Here's how the part is built. I have some questions about the finished solid (model axes, mm). Face numbers are marked on the shaded views. A direction names the side the tool comes from. Round coordinates to 2 decimals unless told otherwise and drop trailing zeros. Order: outer loops, then holes, each group sorted by start corner. A loop starts at its lowest first (then second) coordinate and runs counter-clockwise, first axis right, second up. Notation, with made-up numbers: (76, 33.25) - (128, 33.25) arc R4 ccw to (128, 37.25) - close; hole circle Ø11 at (-28, 18). An arc over 180 degrees is marked (long way). Answer as a JSON object with one key per item and string values.
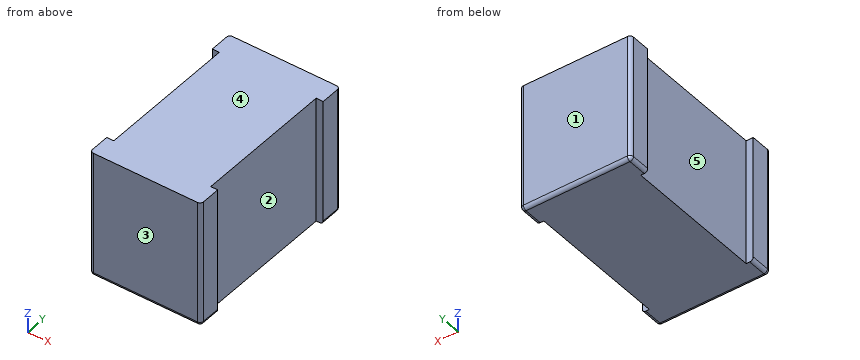
```python
from build123d import *

# Parameters (mm, degrees)
SKETCH_W        = 7.9
SKETCH_H        = 13.2
PAD_DEPTH       = 9.5
SKETCH004_W     = 10
SKETCH004_H     = 9.5
POCKET_DEPTH    = 0.5
POCKET001_DEPTH = 0.5
FILLET001_R     = 0.25


with BuildPart() as part:
    # Sketch → Pad (new body)
    with BuildSketch(Plane.XY):
        Rectangle(SKETCH_W, SKETCH_H)
    extrude(amount=PAD_DEPTH)

    # Sketch004 → Pocket (cut)
    with BuildSketch(Plane.YZ.offset(3.95)):
        with Locations((0, 4.75)):
            Rectangle(SKETCH004_W, SKETCH004_H)
    pocket = extrude(amount=-POCKET_DEPTH, mode=Mode.SUBTRACT)

    # Mirrored: Pocket across YZ
    add(pocket.mirror(Plane.YZ), mode=Mode.SUBTRACT)

    # Sketch005 → Pocket001 (cut)
    with BuildSketch(Plane.XY.offset(9.5)):
        Polygon((-3.95, 6.6), (3.95, 6.6), (3.95, 5), (3.45, 5), (3.45, 0), (-3.45, 0), (-3.45, 5), (-3.95, 5), align=None)
    pocket001 = extrude(amount=-POCKET001_DEPTH, mode=Mode.SUBTRACT)

    # Mirrored001: Pocket001 across XZ
    add(pocket001.mirror(Plane.XZ), mode=Mode.SUBTRACT)

    # Fillet001
    fillet001_edges = [part.edges().sort_by_distance(p)[0] for p in [
        (3.95, -6.6, 4.5),
        (-3.95, -6.6, 4.5),
        (-3.95, 6.6, 4.5),
        (3.95, 6.6, 4.5),
        (0, 6.6, 0),
        (0, -6.6, 0),
        (3.95, -5.8, 0),
        (3.95, 5.8, 0),
        (-3.95, -5.8, 0),
        (-3.95, 5.8, 0),
    ]]
    fillet(fillet001_edges, radius=FILLET001_R)


solid = part.part
```
1. If I drill on L1, parallel to X at y = 4.5, z = 8.5; L2, parallel to Y at x = -3.5, z = 8, over which ranges is the centre line in solid material (lowest first)? Write a range as [from, to].
Responses:
{"L1": "[-3.45, 3.45]", "L2": "[-6.6, -5], [5, 6.6]"}
2. Imagine slicing it at A-A (z = 8). List the corners of the cut face in (x, y) for me, plus the area to 3 significant figures.
Responses:
{"outline": "(-3.95, -6.35) arc R0.25 ccw to (-3.7, -6.6) - (3.7, -6.6) arc R0.25 ccw to (3.95, -6.35) - (3.95, -5) - (3.45, -5) - (3.45, 5) - (3.95, 5) - (3.95, 6.35) arc R0.25 ccw to (3.7, 6.6) - (-3.7, 6.6) arc R0.25 ccw to (-3.95, 6.35) - (-3.95, 5) - (-3.45, 5) - (-3.45, -5) - (-3.95, -5) - close", "area": "94.2 mm2"}
3. Thinking about a two-plate mould opening in Y: for the marked faces 1, 2 and 3, which applies, pulls with the +Y half, pulls with the -Y half, needs draft (parallel to the pull), parting line crosses it, or undercut?
Responses:
{"face 1": "pulls with the +Y half", "face 2": "undercut", "face 3": "pulls with the -Y half"}
4. Imagine slicing it at B-B (y = -3). List the corners of the cut face in (x, z) for me, plus the area to 3 significant figures.
Responses:
{"outline": "(-3.45, 0) - (3.45, 0) - (3.45, 9) - (-3.45, 9) - close", "area": "62.1 mm2"}
5. For P1, Ø2.5, axis at y = -2, z = 4, coming from the +X side; P2, Ø1, axis at y = 1, z = 7, coming from the -X side, each with a flat end and sliding along its axis, tell me the tip position at first contact or that it passes through.
Responses:
{"P1": "x = 3.45", "P2": "x = -3.45"}
6. For the marked faces 4 and 5, which set-ups out of +Z, -Z, +X, -X, +Y, -Y let a thin tool reach every point of the face, with its end or its side?
Responses:
{"face 4": "+Z, +X, -X, +Y, -Y", "face 5": "+Z, -Z, -X"}
